Autodesk Inventor part; units mm, degrees
ref_plane "YZ Plane" through (0, 0, 0) normal (1, 0, 0) x (0, 1, 0)
ref_plane "XZ Plane" through (0, 0, 0) normal (0, 1, 0) x (-1, 0, 0)
ref_plane "XY Plane" through (0, 0, 0) normal (0, 0, 1) x (1, 0, 0)
sketch "Sketch1" plane through (0, 0, 0) normal (0, 1, 0) x (-1, 0, 0)
  line L0 (100, 90) -> (-100, 90)
  line L1 (-100, 90) -> (-100, -90)
  line L2 (-100, -90) -> (100, -90)
  line L3 (100, -90) -> (100, 90)
  point P0 (0, 0)
  point P1 (0, 90)
  point P2 (100, 0)
  dimension "d0" = 200
  dimension "d1" = 180
extrude "Plate1" add sketch "Sketch1" along normal blind 8
sketch "Sketch2" plane through (0, 0, 0) normal (0, -1, 0) x (1, 0, 0)
  line L0 (80, 70) -> (80, -70) construction
  line L1 (-100, -90) -> (-100, 90)
  line L2 (100, 90) -> (100, -90)
  point P0 (0, 0)
  point P1 (80, 0)
  point P2 (-100, 0)
  dimension "d10" = 20
  dimension "d12" = 20
hole "Hole1" at (80, 0, 70) at (80, 0, -70) direction (0, 1, 0) diameter 17 end through all
fillet "Corner Round1" radius 6 4 edges at (100, 4, 90) (100, 4, -90) (-100, 4, -90) (-100, 4, 90)
mirror "Mirror1" about plane through (0, 0, 0) normal (1, 0, 0) of "Hole1"
equation "\"d12\" = d10"
equation "\"d8\" = Thickness"
equation "\"d2\" = Thickness"
equation "\"BendRadius\" = Thickness"
equation "\"BendReliefWidth\" = Thickness"
equation "\"BendReliefDepth\" = 0.5 * Thickness"
equation "\"CornerReliefSize\" = 4 * Thickness"
equation "\"MinimumRemnant\" = 2 * Thickness"
equation "\"TransitionRadius\" = BendRadius"
equation "\"JacobiRadiusSize\" = BendRadius"
equation "\"GapSize\" = Thickness"
properties part number "Сrane plate 6"
Geometry check sheet. Reference: the model listing, model coordinates, mm. Coordinates: 2 decimals unless noted, no trailing zeros. Order: outer loops, then holes, each group sorted by start corner. A loop starts at its lowest first (then second) coordinate and runs counter-clockwise, first axis right, second up. Notation, with made-up numbers: (30, -40) - (74, -40) arc R15 cw to (74, -28) - close; hole circle Ø2 at (42.5, 16.5). An arc over 180 degrees is marked (long way). One line per item, written item: value.
(1) Depth check by flat-ended pin: pin 1 Ø19.5 at (x, z) = (-80, -70) entering from +Y; pin 2 Ø10 at (x, z) = (-80, 70) entering from +Y. Enter the tip coordinate at first touch or a pass-through.
Data:
pin 1: stops at y = 8
pin 2: passes through
(2) Sectioned sample at A-A (x = 80). Enter the section's corners in (y, z), and give its area (3 significant figures).
Data:
outline: (0, -90) - (8, -90) - (8, -78.5) - (0, -78.5) - close; (0, -61.5) - (8, -61.5) - (8, 61.5) - (0, 61.5) - close; (0, 78.5) - (8, 78.5) - (8, 90) - (0, 90) - close
area: 1,170 mm^2
(3) Thickness scan on probe 1 along Z at (x, y) = (-80, 5.25); probe 2 along X at (y, z) = (5.5, -70); probe 3 along X at (y, z) = (6.25, 69). Record the ranges inside material, lowest first. Write a range as from..to.
Data:
probe 1: z = -90..-78.5, -61.5..61.5, 78.5..90
probe 2: x = -100..-88.5, -71.5..71.5, 88.5..100
probe 3: x = -100..-88.44, -71.56..71.56, 88.44..100
(4) Release check for a two-part mould opening along X. For faces 1 (the face through (-80.37, 4.06, -61.51)), 2 (the face through (-80.37, 4.06, 78.49)), 3 (the face through (-98.289, 4.056, 88.196)), 4 (the face through (1, 4, -90)) record: +X half, -X half, draft (parallel to the pull), parting line (faces both ways), or undercut.
Data:
face 1: undercut
face 2: undercut
face 3: -X half
face 4: draft
(5) Sectioned sample at C-C (y = 2.5). Enter the section's corners in (x, z).
Data:
outline: (-100, -84) arc R6 ccw to (-94, -90) - (94, -90) arc R6 ccw to (100, -84) - (100, 84) arc R6 ccw to (94, 90) - (-94, 90) arc R6 ccw to (-100, 84) - close; hole circle Ø17 at (-80, -70); hole circle Ø17 at (-80, 70); hole circle Ø17 at (80, -70); hole circle Ø17 at (80, 70)
(6) Sectioned sample at B-B (z = 70). Enter the section's corners in (x, y).
Data:
outline: (-100, 0) - (-88.5, 0) - (-88.5, 8) - (-100, 8) - close; (-71.5, 0) - (71.5, 0) - (71.5, 8) - (-71.5, 8) - close; (88.5, 0) - (100, 0) - (100, 8) - (88.5, 8) - close
